Input: part model. Units: mm. Frame: model coordinates. A direction names the side the tool comes from. Coordinates: 2 decimals unless noted, no trailing zeros. Loops run counter-clockwise (first coordinate to the right, second up) from the corner with the lowest first, then second, coordinate; pieces in that order, holes last. Notation, with made-up numbers: (29.25, 57) -> (80.25, 57) arc R15 ccw to (80.25, 73) -> close; hole circle Ø3 at (74.5, -2). An arc over 180 degrees is marked (long way). Answer as a JSON object with one key per item and string values.
from build123d import *

# Parameters (mm, degrees)
F1_DEPTH    = 6.35
F2_DEPTH    = 25.4
F3_DEPTH    = 50.8
F4_C1_SIZE2 = 12.7
F4_C1_SIZE  = 7.3323484187
F4_C2_SIZE2 = 12.7
F4_C2_SIZE  = 7.3323484187
F5_SIZE2    = 7.3323484187
F5_SIZE     = 12.7
F6_SIZE2    = 7.3323484187
F6_SIZE     = 12.7
F7_R        = 6.34999


# Not quite as in the source:
# - a fillet or chamfer is up to 0.001 mm smaller than in the source, because OpenCascade refuses the exact size


with BuildPart() as f1:
    # F0 (on Top) → F1 (new body)
    with BuildSketch(Plane.XY):
        Polygon((44.45, 89.8741149127), (-31.75, 89.8741149127), (-31.75, 45.4241149127), (-31.75, -62.5258850873), (44.45, -62.5258850873), align=None)
        Polygon((-25.4, -56.1758850873), (-25.4, 45.4241149127), (-25.4, 83.5241149127), (6.35, 83.5241149127), (38.1, 83.5241149127), (38.1, -18.0758850873), (38.1, -56.1758850873), (6.35, -56.1758850873), align=None, mode=Mode.SUBTRACT)
    extrude(amount=F1_DEPTH)

    # F0 (on Top) → F2 (join)
    with BuildSketch(Plane.XY):
        with BuildLine():
            Line((-6.35, 45.4241149127), (-25.4, 45.4241149127))
            Line((-25.4, 45.4241149127), (-25.4, -56.1758850873))
            Line((-25.4, -56.1758850873), (6.35, -56.1758850873))
            Line((6.35, -56.1758850873), (6.35, -30.7758850873))
            ThreePointArc((6.35, -30.7758850873), (10.0697438789, -21.7956289662), (19.05, -18.0758850873))
            Line((19.05, -18.0758850873), (38.1, -18.0758850873))
            Line((38.1, -18.0758850873), (38.1, 83.5241149127))
            Line((38.1, 83.5241149127), (6.35, 83.5241149127))
            Line((6.35, 83.5241149127), (6.35, 58.1241149127))
            ThreePointArc((6.35, 58.1241149127), (2.6302561211, 49.1438587917), (-6.35, 45.4241149127))
        make_face()
    extrude(amount=F2_DEPTH)

    # F0 (on Top) → F3 (join)
    with BuildSketch(Plane.XY):
        with BuildLine():
            Line((-25.4, 83.5241149127), (-25.4, 45.4241149127))
            Line((-25.4, 45.4241149127), (-6.35, 45.4241149127))
            ThreePointArc((-6.35, 45.4241149127), (2.6302561211, 49.1438587917), (6.35, 58.1241149127))
            Line((6.35, 58.1241149127), (6.35, 83.5241149127))
            Line((6.35, 83.5241149127), (-25.4, 83.5241149127))
        make_face()
        with BuildLine():
            Line((6.35, -30.7758850873), (6.35, -56.1758850873))
            Line((6.35, -56.1758850873), (38.1, -56.1758850873))
            Line((38.1, -56.1758850873), (38.1, -18.0758850873))
            Line((38.1, -18.0758850873), (19.05, -18.0758850873))
            ThreePointArc((19.05, -18.0758850873), (10.0697438789, -21.7956289662), (6.35, -30.7758850873))
        make_face()
    extrude(amount=F3_DEPTH)

    # F4: chamfer of 12.7 x 7.3323484187 on 2 edges, made by hand

    # F4_c1
    f4_c1_edges = [f1.edges().sort_by_distance(p)[0] for p in [
        (-9.525, 83.5241149127, 50.8),
    ]]
    f4_c1_side = f1.faces().sort_by_distance((-9.525, 83.3774679444, 50.8))[0]
    chamfer(f4_c1_edges, length=F4_C1_SIZE, length2=F4_C1_SIZE2, reference=f4_c1_side)

    # F4_c2
    f4_c2_edges = [f1.edges().sort_by_distance(p)[0] for p in [
        (-25.4, 60.8079407034, 50.8),
    ]]
    f4_c2_side = f1.faces().sort_by_distance((-25.2533530316, 60.8079407034, 50.8))[0]
    chamfer(f4_c2_edges, length=F4_C2_SIZE, length2=F4_C2_SIZE2, reference=f4_c2_side)

    # F5
    f5_edges = [f1.edges().sort_by_distance(p)[0] for p in [
        (38.1, -37.125885, 50.8),
        (22.225, -56.175885, 50.8),
    ]]
    chamfer(f5_edges, length=F5_SIZE, length2=F5_SIZE2)

    # F6
    f6_edges = [f1.edges().sort_by_distance(p)[0] for p in [
        (-25.4, -5.375885, 25.4),
        (-9.525, -56.175885, 25.4),
        (38.1, 32.724115, 25.4),
        (22.225, 83.524115, 25.4),
    ]]
    f6_side = f1.faces().sort_by_distance((6.35, 13.674115, 25.4))[0]
    chamfer(f6_edges, length=F6_SIZE, length2=F6_SIZE2, reference=f6_side)

    # F7 (radius 6.35 in the source; OpenCascade refuses exactly that, so slightly less here)
    f7_edges = [f1.edges().sort_by_distance(p)[0] for p in [
        (44.45, 13.674115, 6.35),
        (6.35, -62.525885, 6.35),
        (-31.75, 13.674115, 6.35),
        (6.35, 89.874115, 6.35),
    ]]
    fillet(f7_edges, radius=F7_R)


solid = f1.part
1. Section query A-A (z = 31.5). Return loops of the section in (x, y), plus the area to 3 significant figures.
Reply:
{"outline": "(-25.4, 45.42) -> (-6.35, 45.42) arc R12.7 ccw to (6.35, 58.12) -> (6.35, 83.52) -> (-25.4, 83.52) -> close; (6.35, -56.18) -> (38.1, -56.18) -> (38.1, -18.08) -> (19.05, -18.08) arc R12.7 ccw to (6.35, -30.78) -> close", "area": "2,350 mm2"}
2. Pin query (flat end, axial travel): P1, Ø21, axis at x = -12.5, z = 28, coming from the -Y side; P2, Ø1.5, axis at x = 16, y = 59.5, coming from the +Z side; P3, Ø8, axis at y = -15, z = 21.5, coming from the -X side. Return the tip coordinate at first contact, or that it passes through.
Reply:
{"P1": "stops at y = -56.18", "P2": "stops at z = 25.4", "P3": "stops at x = -25.4"}
3. Line query: line 1 along Z through (x, y) = (21.5, 60.5); line 2 along X through (y, z) = (-26, 7.5); line 3 along Y through (x, z) = (24, 25.5). Output: solid intervals per line, ascending.
Reply:
{"line 1": "z = 0 to 25.4", "line 2": "x = -25.4 to 38.1", "line 3": "y = -56.18 to -18.08"}
4. Access query for faces 1 (the face through (6, 14, 25.4)), 2 (the face through (-19.14, -4.66, 21.68)), 3 (the face through (-25.4, 30, 15)), 4 (the face through (38.1, -3, 15)), 5 (the face through (18.919, 77.263, 21.682)). Directions: +Z, -Z, +X, -X, +Y, -Y. A direction counts if a zero-diameter tool reaches every point of the face in a straight line with its end or side. Return the directions, or none.
Reply:
{"face 1": "+Z", "face 2": "+Z, -X, -Y", "face 3": "+Z, -X, +Y, -Y", "face 4": "+Z, +X, +Y, -Y", "face 5": "+Z, +X, +Y"}
5. Section query D-D (z = 20.5). Return loops of the section in (x, y), plus the area to 3 significant figures.
Reply:
{"outline": "(-25.4, 45.42) -> (-21.19, 45.42) -> (-21.19, -51.96) -> (6.35, -51.96) -> (6.35, -56.18) -> (38.1, -56.18) -> (38.1, -18.08) -> (33.89, -18.08) -> (33.89, 79.31) -> (6.35, 79.31) -> (6.35, 83.52) -> (-25.4, 83.52) -> close", "area": "7,780 mm2"}
